For this review, take the finished solid that the model builds, in its own axes (mm). A direction names the side the tool comes from. Round coordinates to 2 decimals unless told otherwise and drop trailing zeros. Order: outer loops, then holes, each group sorted by start corner. A loop starts at its lowest first (then second) coordinate and runs counter-clockwise, first axis right, second up. Notation, with made-up numbers: (0, 7.5) - (21, 7.5) arc R9 ccw to (21, 11.5) - close; hole circle Ø10 at (-14.75, 6.5). An arc over 180 degrees is marked (long way). One line per item, written item: value.
Autodesk Inventor part; units mm, degrees
ref_plane "Start Plane" through (0, 0, 16.9601) normal (0, 0, 1) x (1, 0, 0)
ref_plane "End Plane" through (0, 0, 375.4098) normal (0, 0, 1) x (1, 0, 0)
ref_plane "Work Plane5" through (1020.9815, 716.9447, 401.9181) normal (-0.0261419, -0.0006839, 0.999658) x (0.9996582, -0.0000089, 0.0261419)
ref_plane "Start Plane" through (0, 0, 16.9601) normal (0, 0, 1) x (1, 0, 0)
ref_plane "End Plane" through (0, 0, 375.4098) normal (0, 0, 1) x (1, 0, 0)
sketch "Sketch" plane through (0, 0, 0) normal (0, 0, 1) x (1, 0, 0)
  line L0 (25.4, 0) -> (0, 0)
  line L1 (0, 0) -> (0, 25.4)
  line L2 (0, 25.4) -> (1.651, 25.4)
  line L3 (3.175, 23.876) -> (3.175, 6.477)
  line L4 (6.477, 3.175) -> (23.876, 3.175)
  line L5 (25.4, 1.651) -> (25.4, 0)
  line L6 (0, -11.0414) -> (0, 31.5385) construction
  line L7 (-11.0414, 0) -> (31.5385, 0) construction
  arc A0 (3.175, 6.477) -> (6.477, 3.175) centre (6.477, 6.477) ccw
  arc A1 (3.175, 23.876) -> (1.651, 25.4) centre (1.651, 23.876) ccw
  arc A2 (25.4, 1.651) -> (23.876, 3.175) centre (23.876, 1.651) ccw
  line L8 (0, 40.0545) -> (0, -19.5574) construction
  line L9 (-19.5574, 0) -> (40.0545, 0) construction
  point P0 (3.175, 25.4)
  point P1 (3.175, 3.175)
  point P2 (25.4, 3.175)
  dimension "d0" = 25.4
  dimension "d1" = 25.4
  dimension "d2" = 3.175
  dimension "d3" = 3.175
  dimension "d10" = 0
  dimension "d11" = 0
  dimension "d14" = 3.302
  dimension "d15" = 1.524
extrude "Body" add sketch "Sketch" along normal up to surface (358.4496 mm away) from surface at 16.9601
sketch "Sketch3" plane through (0, 0, 0) normal (0, 0, 1) x (1, 0, 0)
  line L0 (0, 0) -> (10, 0)
ref_plane "Work Plane3" through (0, 0, 0) normal (0, -1, 0) x (1, 0, 0)
ref_plane "Work Plane5" through (1020.9815, 716.9447, 401.9181) normal (-0.0261419, -0.0006839, 0.999658) x (0.9996582, -0.0000089, 0.0261419)
split "Split2" plane through (1020.9815, 716.9447, 401.9181) removes the side toward (-0.0261419, -0.0006839, 0.999658)
ref_plane "Work Plane6" through (-4.5304, 249.7362, -76.5277) normal (0.034189, -0.3838526, -0.9227612) x (0.9848666, 0.1699087, -0.034189)
split "Split3" plane through (-4.5304, 249.7362, -76.5277) removes the side toward (0.034189, -0.3838526, -0.9227612)
sketch "Sketch4" plane through (0, 0, 0) normal (0, -1, 0) x (1, 0, 0)
  line L0 (-2, 16.9601) -> (12, 16.9601)
  line L1 (-2, 375.4098) -> (12, 375.4098)
  dimension "d17" = 358.4496
equation "\"d0\" = G_H"
equation "\"d1\" = G_H"
equation "\"d2\" = G_T"
equation "\"d3\" = G_T"
equation "\"d14\" = G_IR"
equation "\"d15\" = G_ER"
equation "\"d4\" = G_L"
equation "\"G_H\" = 25.4"
equation "\"G_T\" = 3.175"
equation "\"G_ER\" = 1.524"
equation "\"G_IR\" = 3.302"
equation "\"G_L\" = 358.43341"
equation "\"ex\" = 0"
equation "\"G_OFFSET_START\" = -16.96012"
equation "\"G_OFFSET_END\" = -24.72708"
equation "\"d12\" = -G_OFFSET_START"
equation "\"d13\" = G_OFFSET_END + B_L"
equation "\"B_L\" = 400.13684"
properties part number "AISC - L 1 x 1 x 1/8 - 14.112" material "Steel, Mild"
Item 1: For P1, Ø8, axis at y = 21.5, z = 64, coming from the +X side (3 decimals); P2, Ø5, axis at x = 17.5, y = 3, coming from the +Z side, all flat-tipped, find the tip position at first contact; note any pin that passes through.
Returned:
P1: x = 3.175
P2: z = 375.25
Item 2: Take a section at A-A (z = 242.5). Write out the cut boundary in (x, y) (3 decimals).
Returned:
outline: (0, 0) - (25.4, 0) - (25.4, 1.651) arc R1.524 ccw to (23.876, 3.175) - (6.477, 3.175) arc R3.302 cw to (3.175, 6.477) - (3.175, 23.876) arc R1.524 ccw to (1.651, 25.4) - (0, 25.4) - close
Item 3: Wall thickness on line 1 (X direction, y = 21, z = 318) (3 decimals); line 2 (Y direction, x = 2, z = 164); line 3 (X direction, y = 1.75, z = 136.5): over which ranges is each line inside the solid? List them lowest first.
Returned:
line 1: 0 to 3.175
line 2: 0 to 25.36
line 3: 0 to 25.4
Item 4: Take a section at B-B (y = 16.25). Write out the cut boundary in (x, z) (3 decimals), plus the area to 3 significant figures.
Returned:
outline: (0, 20.766) - (3.175, 20.884) - (3.175, 374.822) - (0, 374.739) - close
area: 1,120 mm^2
Item 5: Machinability: for faces 1 (the flat face through (15, 3.175, 198)), 2 (the flat face through (13, 0, 199)), which of the approach directions +Z, -Z, +X, -X, +Y, -Y give a long, thin tool a straight path to every point of the face, cutting with its end or side? Answer none if there is none.
Returned:
face 1: +Z, -Z, +X, +Y
face 2: +Z, -Z, +X, -X, -Y
Item 6: Take a section at C-C (x = 14.5). Write out the cut boundary in (y, z) (3 decimals).
Returned:
outline: (0, 28.063) - (3.175, 26.743) - (3.175, 375.109) - (0, 375.107) - close
